Geometry check sheet. Reference: drawing and pictorial views, mm from the part's lowest x, y, z. Give positions to 0.01 mm unless a question says otherwise; leave off trailing zeros. Write each loop counter-clockwise with the first axis right and the second up, starting at its lowest first coordinate (ties: lowest second). Pieces come first, ordered by that corner, then holes. Notation, with made-up numbers: M 33,73.25 L 82,73.25 A23 cw 82,104.25 Z; hole C 89,59 d1. An arc over 180 degrees is marked long. One line per item, written item: value. Start each with the question number.
1. Release check for a two-part mould opening along Y. For the marked faces 1, 2 and 3 record: pulls with the +Y half, pulls with the -Y half, needs draft (parallel to the pull), parting line crosses it, or undercut.
2. Cross-section at A-A on x = 26. Record the cut outline in (y, z), then the cut area to 3 significant figures.
3. Cross-section at B-B on y = 26. Record the cut outline in (x, z), then the cut area to 3 significant figures.
4. Gauge pin test, flat ends, axial feed: pin 1 (1.5 mm diameter, centred on x = 34.5, z = 4.5, fed in from +Y); pin 2 (3 mm diameter, centred on x = 27, y = 38.5, fed in from -Z); pin 3 (1.5 mm diameter, centred on y = 27, z = 5.5, fed in from +X); pin 4 (1.5 mm diameter, centred on x = 36, z = 4.5, fed in from -Y). Record the tip position at first contact, or that the pin passes through.
5. Cross-section at D-D on z = 1.25. Record the cut outline in (x, y).
6. Cross-section at C-C on z = 4.5. Record the cut outline in (x, y), then the cut area to 3 significant figures.
7. Scan lines: line 1 (Z direction, x = 16, y = 45.5); line 2 (Y direction, x = 25.5, z = 0.5); line 3 (X direction, y = 17.5, z = 5.25). Record each from-to range of solid material in increasing order.
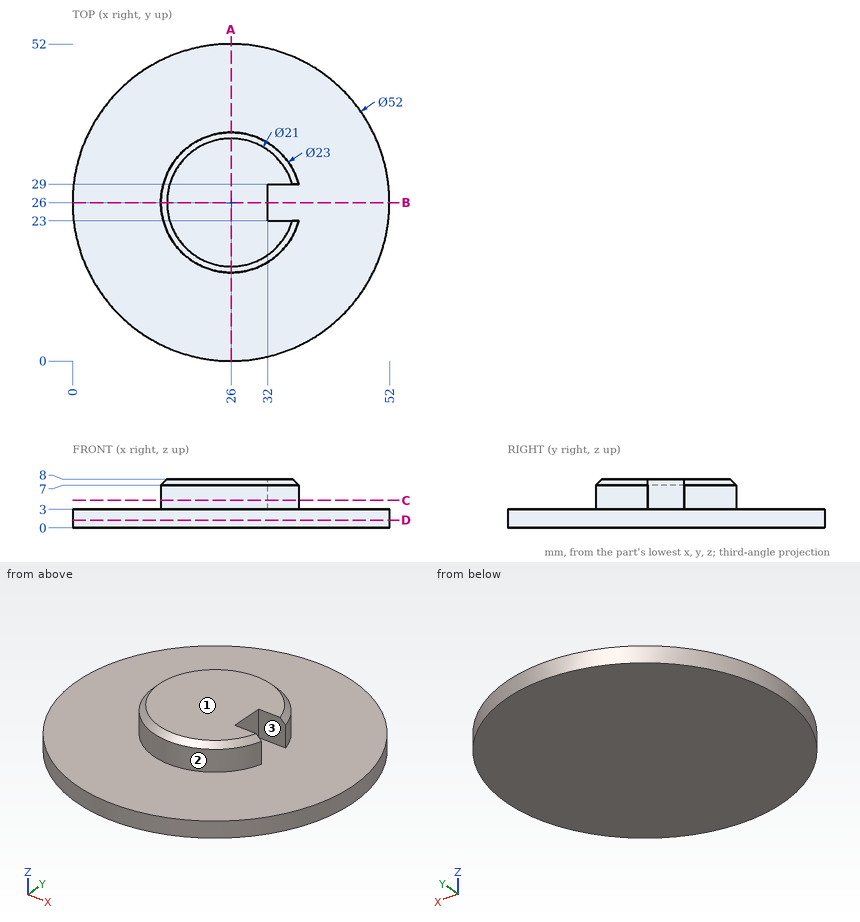
Report:
1. face 1: needs draft
1. face 2: parting line crosses it
1. face 3: undercut
2. outline: M 0,0 L 52,0 L 52,3 L 37.5,3 L 37.5,7 L 36.5,8 L 15.5,8 L 14.5,7 L 14.5,3 L 0,3 Z
2. area: 270 mm^2
3. outline: M 0,0 L 52,0 L 52,3 L 32,3 L 32,8 L 15.5,8 L 14.5,7 L 14.5,3 L 0,3 Z
3. area: 243 mm^2
4. pin 1: stops at y = 34.5
4. pin 2: stops at z = 0
4. pin 3: stops at x = 32
4. pin 4: stops at y = 19.17
5. outline: C 26,26 d52
6. outline: M 32,23 L 32,29 L 37.1,29 A11.5 ccw long 37.1,23 Z
6. area: 383 mm^2
7. line 1: z = 0 to 3
7. line 2: y = 0 to 52
7. line 3: x = 18.25 to 33.75
